The listing builds one solid part. Answer for the finished solid, in the listing's coordinates (mm). Face numbers are marked on the shaded views. Round coordinates to 2 decimals unless told otherwise and drop trailing zeros. Loops run counter-clockwise (first coordinate to the right, second up) from the corner with the lowest first, then second, coordinate; pieces in that order, holes last. Notation, with made-up numbers: M 52.25,40 L 67.25,40 A24 ccw 67.25,67 Z; hole C 23,53.25 d1. An arc over 180 degrees is marked long. Answer as a JSON object with one key per item and string values.
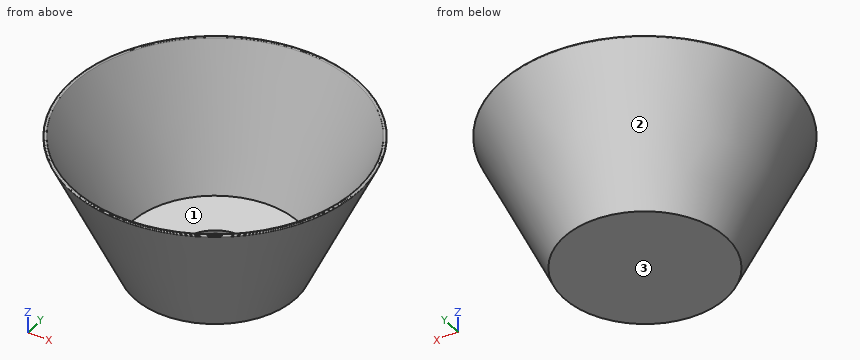
```python
from build123d import *

# Parameters (mm, degrees)
F0_R     = 47
F1_DEPTH = 79
F1_TAPER = -25
F2_R     = 82
F3_DEPTH = 71
F3_TAPER = 25
F4_R     = 20
F5_DEPTH = 2
F6_R     = 0.5


with BuildPart() as f1:
    # F0 (on Top) → F1 (new body)
    with BuildSketch(Plane.XY):
        Circle(F0_R)
    extrude(amount=F1_DEPTH, taper=F1_TAPER)

    # F2 (on face) → F3 (cut)
    with BuildSketch(Plane.XY.offset(79)):
        Circle(F2_R)
    extrude(amount=-F3_DEPTH, taper=F3_TAPER, mode=Mode.SUBTRACT)

    # F4 (on face) → F5 (cut)
    with BuildSketch(Plane.XY.offset(8)):
        Circle(F4_R)
    extrude(amount=-F5_DEPTH, mode=Mode.SUBTRACT)

    # F6
    f6_edges = [f1.edges().sort_by_distance(p)[0] for p in [
        (-83.838305, 0, 79),
        (-82, 0, 79),
    ]]
    fillet(f6_edges, radius=F6_R)


solid = f1.part
```
Item 1: The part is cut by section A-A (x = 0). Give the vertices of the cut face in (y, z).
Values follow:
{"outline": "M -83.51,78.29 L -47,0 L 47,0 L 83.51,78.29 A0.5 ccw 83.05,79 L 82.32,79 A0.5 ccw 81.87,78.71 L 48.89,8 L 20,8 L 20,6 L -20,6 L -20,8 L -48.89,8 L -81.87,78.71 A0.5 ccw -82.32,79 L -83.05,79 A0.5 ccw Z"}
Item 2: The part is cut by section C-C (z = 60). Give the vertices of the cut face in (x, y).
Values follow:
{"outline": "C 0,0 d149.96; hole C 0,0 d146.28"}
Item 3: The part is cut by section B-B (z = 41). Give the vertices of the cut face in (x, y).
Values follow:
{"outline": "C 0,0 d132.24; hole C 0,0 d128.56"}
Item 4: Flat-ended cylindrical pins translate along their axes: P1, Ø12, axis at x = 6, y = 6.5, coming from the +Z side; P2, Ø6, axis at x = 23, y = -9.5, coming from the -Z side; P3, Ø8, axis at x = 65.5, z = 63.5, coming from the -Y side; P4, Ø1, axis at y = -24.5, z = 27, coming from the +X side. Find the tip coordinate at first contact, or state that the pin passes through.
Values follow:
{"P1": "z = 6", "P2": "z = 0", "P3": "y = -46.52", "P4": "x = 54.66"}
Item 5: Straight lines are drawn through the part: line 1 (X direction, y = 58, z = 64); line 2 (X direction, y = -24, z = 35); line 3 (Y direction, x = 0, z = 7.4). For each, find the intervals that lie inside material, in ascending order.
Values follow:
{"line 1": "-50.41 to -47.56, 47.56 to 50.41", "line 2": "-58.6 to -56.6, 56.6 to 58.6", "line 3": "-50.45 to -20, 20 to 50.45"}
Item 6: Determine the mould class of the marked faces 1, 2 and 3 for opening direction X: released by +X, released by -X, zero draft, split by the parting line, or undercut.
Values follow:
{"face 1": "undercut", "face 2": "split by the parting line", "face 3": "zero draft"}
